```python
from build123d import *

# Parameters (mm, degrees)
EXTRUDE_1_DEPTH        = 3
SKETCH_2_R             = 1.25
CUT_EXTRUDE_1_DEPTH    = 6
SKETCH_3_R             = 1.25
CUT_EXTRUDE_2_DEPTH    = 3
HOLE_WIZARD_M3_1_D     = 2.5
HOLE_WIZARD_M3_1_DEPTH = 4.5
HOLE_WIZARD_M3_1_TIP   = 0.721687836
CHAMFER_1_SIZE         = 0.2
CHAMFER_2_SIZE         = 0.2


with BuildPart() as part:
    # 草图1 → 凸台-拉伸1 (new body, symmetric)
    with BuildSketch(Plane.XY):
        Polygon((0, 17), (0, 0), (12, 0), (12, 5), (5, 5), (5, 17), align=None)
    extrude(amount=EXTRUDE_1_DEPTH, both=True)

    # 草图2 → 切除-拉伸1 (cut)
    with BuildSketch(Plane(origin=(5, 0, 0), x_dir=(0, 0, -1), z_dir=(1, 0, 0))):
        with Locations((0, 14)):
            Circle(SKETCH_2_R)
        with Locations((0, 8)):
            Circle(SKETCH_2_R)
    extrude(amount=-CUT_EXTRUDE_1_DEPTH, mode=Mode.SUBTRACT)

    # 草图3 → 切除-拉伸2 (cut)
    with BuildSketch(Plane.XZ):
        with Locations((9, 0)):
            Circle(SKETCH_3_R)
        with Locations((3, 0)):
            Circle(SKETCH_3_R)
    extrude(amount=-CUT_EXTRUDE_2_DEPTH, mode=Mode.SUBTRACT)

    # M3 螺纹孔1
    with Locations(Plane(origin=(3, 0, 0), x_dir=(0, 0, -1), z_dir=(0, -1, 0))):
        with Locations((0, 0), (0, 6)):
            Hole(HOLE_WIZARD_M3_1_D / 2, depth=HOLE_WIZARD_M3_1_DEPTH)
            with Locations((0, 0, -(HOLE_WIZARD_M3_1_DEPTH + HOLE_WIZARD_M3_1_TIP / 2))):  # 120° drill point
                Cone(0, HOLE_WIZARD_M3_1_D / 2, HOLE_WIZARD_M3_1_TIP, mode=Mode.SUBTRACT)

    # 倒角1
    chamfer_1_edges = [part.edges().sort_by_distance(p)[0] for p in [
        (6, 0, 3),
        (5, 17, 0),
        (12, 5, 0),
        (12, 0, 0),
        (0, 17, 0),
        (12, 2.5, 3),
        (8.5, 5, 3),
        (5, 11, 3),
        (2.5, 17, 3),
        (5, 11, -3),
        (8.5, 5, -3),
        (12, 2.5, -3),
        (0, 8.5, 3),
        (6, 0, -3),
        (0, 8.5, -3),
        (2.5, 17, -3),
    ]]
    chamfer(chamfer_1_edges, length=CHAMFER_1_SIZE)

    # 倒角2
    chamfer_2_edges = [part.edges().sort_by_distance(p)[0] for p in [
        (0, 0, 0),
    ]]
    chamfer(chamfer_2_edges, length=CHAMFER_2_SIZE)


solid = part.part
```
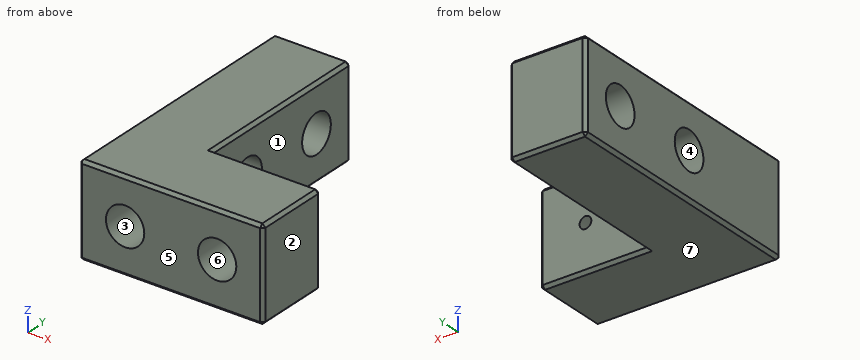
Geometry: final body of the model. Coordinates: model frame, mm. Face numbers are marked on the shaded views. A direction names the side the tool comes from. Round coordinates to 2 decimals unless told otherwise and drop trailing zeros. Loops run counter-clockwise (first coordinate to the right, second up) from the corner with the lowest first, then second, coordinate; pieces in that order, holes last.
Item 1: Line query: L1, parallel to Y at x = 1.1, z = 0; L2, parallel to X at y = 2.15, z = 0; L3, parallel to Z at x = 3, y = 1.5. Output: solid intervals per line, ascending.
Checked values:
L1: y = 0 to 6.75, 9.25 to 12.75, 15.25 to 17
L2: x = 0 to 1.75, 4.25 to 7.75, 10.25 to 12
L3: z = -3 to -1.25, 1.25 to 3
Item 2: Section A-A, the plane y = 8. Output: boundary loops of the cut face in (x, z), plus the area to 3 significant figures.
Checked values:
outline: (0, -2.8) - (0.2, -3) - (4.8, -3) - (5, -2.8) - (5, -1.25) - (0, -1.25) - close; (0, 1.25) - (5, 1.25) - (5, 2.8) - (4.8, 3) - (0.2, 3) - (0, 2.8) - close
area: 17.4 mm2
Item 3: Section D-D, the plane x = 9. Output: boundary loops of the cut face in (y, z), plus the area to 3 significant figures.
Checked values:
outline: (0, -2.8) - (0.2, -3) - (4.8, -3) - (5, -2.8) - (5, -0.38) - (4.5, -1.25) - (0, -1.25) - close; (0, 1.25) - (4.5, 1.25) - (5, 0.38) - (5, 2.8) - (4.8, 3) - (0.2, 3) - (0, 2.8) - close
area: 17.9 mm2
Item 4: Section B-B, the plane x = 1. Output: boundary loops of the cut face in (y, z).
Checked values:
outline: (0, -2.8) - (0.2, -3) - (16.8, -3) - (17, -2.8) - (17, 2.8) - (16.8, 3) - (0.2, 3) - (0, 2.8) - close; hole circle Ø2.5 at (8, 0); hole circle Ø2.5 at (14, 0)
Item 5: Section C-C, the plane y = 11. Output: boundary loops of the cut face in (x, z), plus the area to 3 significant figures.
Checked values:
outline: (0, -2.8) - (0.2, -3) - (4.8, -3) - (5, -2.8) - (5, 2.8) - (4.8, 3) - (0.2, 3) - (0, 2.8) - close
area: 29.9 mm2
Item 6: Mould query, pull axis Z, two halves, no side actions, for the marked faces 4, 5, 6 and 7. Classes: released by +Z, released by -Z, zero draft, split by the parting line, or undercut.
Checked values:
face 4: undercut
face 5: zero draft
face 6: undercut
face 7: released by -Z
Item 7: Reachability of the marked faces 1, 2 and 3 from +Z, -Z, +X, -X, +Y, -Y: full face, straight path, thin tool, end or side. Return the list, or none.
Checked values:
face 1: +Z, -Z, +X, +Y
face 2: +Z, -Z, +X, +Y, -Y
face 3: -Y
Item 8: Contact query for flat-ended pins moving along their axis: P1, Ø3, axis at x = 9, z = 0, coming from the +Y side; P2, Ø3, axis at y = 14, z = 0, coming from the +X side. Output: stop coordinate, or through.
Checked values:
P1: stops at y = 5
P2: stops at x = 5
